Read the model definition and answer for the solid it produces. Units are mm, in the model's axes. A direction names the side the tool comes from. Give positions to 0.01 mm unless a question says otherwise; leave off trailing zeros. Loops run counter-clockwise (first coordinate to the right, second up) from the corner with the lowest first, then second, coordinate; pieces in that order, holes last.
(1) Find section D-D, the plane x = -87. Write down the section's boundary in (y, z), then the cut area to 3 significant figures.
(2) Find section A-A, the plane y = 90.5. Write down the section's boundary in (x, z), then the cut area to 3 significant figures.
(3) Each of these flat-tipped pins is pushed along its axis until it touches: P1, Ø3, axis at x = -18.28, y = 0, coming from the +Z side; P2, Ø0.7, axis at x = -12.5, z = 44.5, coming from the +Y side (3 decimals). Where does it stop, or does it pass through?
(4) Find section B-B, the plane x = 1. Write down the section's boundary in (y, z) (3 decimals), then the cut area to 3 significant figures.
(5) Find section C-C, the plane z = 45.65. State how many separate pieces and enclosed holes the cut face has, then the cut area to 3 significant figures.
(6) Which of the six approach directions +Z, -Z, +X, -X, +Y, -Y give full straight-line access (tool end or side, diameter ignored) to faces 1 (the face through (-38.53, 74.84, 44.87)), 2 (the face through (-35, 2, 43.676)), 3 (the face through (38.53, -74.84, 44.87))?
(7) Straight lines are drawn through the part: probe 1 along Y at (x, z) = (15.24, 44.3) (3 decimals); probe 2 along X at (y, z) = (20, 45.15); probe 3 along Y at (x, z) = (-27, 43.8) (3 decimals). For each, find the intervals that lie inside material, in ascending order.
```python
from build123d import *

# Parameters (mm, degrees)
SKETCH_R        = 2.3622
SKETCH_R_2      = 17.78
PAD_DEPTH       = 2.3622
FILLET_R        = 6.35
FILLET001_R     = 6.35
FILLET002_R     = 6.35
FILLET003_R     = 6.35
FILLET004_R     = 6.35
FILLET005_R     = 3.175
FILLET006_R     = 3.175
FILLET007_R     = 6.35
FILLET008_R     = 6.35
FILLET009_R     = 6.35
FILLET010_R     = 6.35
FILLET011_R     = 6.35
FILLET012_R     = 3.175
FILLET013_R     = 3.175
SKETCH001_R     = 1.651
POCKET_DEPTH    = 2.3632
SKETCH002_R     = 2.2479
POCKET001_DEPTH = 2.3632
SKETCH003_R     = 2.2479
POCKET002_DEPTH = 4.99999


with BuildPart() as part:
    # Sketch (on DatumPlane) → Pad (new body)
    with BuildSketch(Plane.XY.offset(43.6758)):
        Polygon((40.4368, 73.025), (-40.4368, 73.025), (-40.4368, 127), (-65.8368, 127), (-197.6882, 22.225), (-197.6882, -22.225), (-65.8368, -127), (-40.4368, -127), (-40.4368, -73.025), (40.4368, -73.025), (40.4368, -127), (72.1868, -127), (72.1868, 127), (40.4368, 127), align=None)
        with Locations((-21.3868, 66.675)):
            Circle(SKETCH_R, mode=Mode.SUBTRACT)
        with Locations((-21.3868, 53.975)):
            Circle(SKETCH_R, mode=Mode.SUBTRACT)
        with Locations((-21.3868, -53.975)):
            Circle(SKETCH_R, mode=Mode.SUBTRACT)
        with Locations((-21.3868, -66.675)):
            Circle(SKETCH_R, mode=Mode.SUBTRACT)
        with Locations((15.0368, 66.675)):
            Circle(SKETCH_R, mode=Mode.SUBTRACT)
        with Locations((15.24, 53.975)):
            Circle(SKETCH_R, mode=Mode.SUBTRACT)
        with Locations((15.24, -53.975)):
            Circle(SKETCH_R, mode=Mode.SUBTRACT)
        with Locations((15.24, -66.675)):
            Circle(SKETCH_R, mode=Mode.SUBTRACT)
        with Locations((-165.9382, 0)):
            Circle(SKETCH_R_2, mode=Mode.SUBTRACT)
    extrude(amount=PAD_DEPTH)

    # Fillet
    fillet_edges = [part.edges().sort_by_distance(p)[0] for p in [
        (-197.6882, -22.225, 44.8569),
    ]]
    fillet(fillet_edges, radius=FILLET_R)

    # Fillet001
    fillet001_edges = [part.edges().sort_by_distance(p)[0] for p in [
        (-65.8368, -127, 44.8569),
    ]]
    fillet(fillet001_edges, radius=FILLET001_R)

    # Fillet002
    fillet002_edges = [part.edges().sort_by_distance(p)[0] for p in [
        (-40.4368, -127, 44.8569),
    ]]
    fillet(fillet002_edges, radius=FILLET002_R)

    # Fillet003
    fillet003_edges = [part.edges().sort_by_distance(p)[0] for p in [
        (-40.4368, -73.025, 44.8569),
    ]]
    fillet(fillet003_edges, radius=FILLET003_R)

    # Fillet004
    fillet004_edges = [part.edges().sort_by_distance(p)[0] for p in [
        (40.4368, -73.025, 44.8569),
    ]]
    fillet(fillet004_edges, radius=FILLET004_R)

    # Fillet005
    fillet005_edges = [part.edges().sort_by_distance(p)[0] for p in [
        (40.4368, -127, 44.8569),
    ]]
    fillet(fillet005_edges, radius=FILLET005_R)

    # Fillet006
    fillet006_edges = [part.edges().sort_by_distance(p)[0] for p in [
        (72.1868, -127, 44.8569),
    ]]
    fillet(fillet006_edges, radius=FILLET006_R)

    # Fillet007
    fillet007_edges = [part.edges().sort_by_distance(p)[0] for p in [
        (-197.6882, 22.225, 44.8569),
    ]]
    fillet(fillet007_edges, radius=FILLET007_R)

    # Fillet008
    fillet008_edges = [part.edges().sort_by_distance(p)[0] for p in [
        (-65.8368, 127, 44.8569),
    ]]
    fillet(fillet008_edges, radius=FILLET008_R)

    # Fillet009
    fillet009_edges = [part.edges().sort_by_distance(p)[0] for p in [
        (-40.4368, 127, 44.8569),
    ]]
    fillet(fillet009_edges, radius=FILLET009_R)

    # Fillet010
    fillet010_edges = [part.edges().sort_by_distance(p)[0] for p in [
        (40.4368, 73.025, 44.8569),
    ]]
    fillet(fillet010_edges, radius=FILLET010_R)

    # Fillet011
    fillet011_edges = [part.edges().sort_by_distance(p)[0] for p in [
        (-40.4368, 73.025, 44.8569),
    ]]
    fillet(fillet011_edges, radius=FILLET011_R)

    # Fillet012
    fillet012_edges = [part.edges().sort_by_distance(p)[0] for p in [
        (40.4368, 127, 44.8569),
    ]]
    fillet(fillet012_edges, radius=FILLET012_R)

    # Fillet013
    fillet013_edges = [part.edges().sort_by_distance(p)[0] for p in [
        (72.1868, 127, 44.8569),
    ]]
    fillet(fillet013_edges, radius=FILLET013_R)

    # Sketch001 (on Face39 of Fillet013) → Pocket (cut, through all)
    with BuildSketch(Plane.XY.offset(46.038)):
        with Locations((-26.2382, 0)):
            Circle(SKETCH001_R)
        with Locations((-34.2011, 0)):
            Circle(SKETCH001_R)
        with Locations((-26.2382, 9.525)):
            Circle(SKETCH001_R)
        with Locations((-18.2753, 0)):
            Circle(SKETCH001_R)
        with Locations((-26.2382, -9.525)):
            Circle(SKETCH001_R)
    extrude(amount=-POCKET_DEPTH, mode=Mode.SUBTRACT)

    # Sketch002 (on Face44 of Pocket) → Pocket001 (cut, through all)
    with BuildSketch(Plane.XY.offset(46.038)):
        with Locations((-96.923253, -96.214243)):
            Circle(SKETCH002_R)
        with Locations((-72.065864, -115.967033)):
            Circle(SKETCH002_R)
        with Locations((-72.065864, 115.967033)):
            Circle(SKETCH002_R)
        with Locations((-96.923253, 96.214243)):
            Circle(SKETCH002_R)
    extrude(amount=-POCKET001_DEPTH, mode=Mode.SUBTRACT)

    # Sketch003 (on Face48 of Pocket001) → Pocket002 (cut)
    with BuildSketch(Plane.XY.offset(46.038)):
        with Locations((67.4243, -117.475)):
            Circle(SKETCH003_R)
        with Locations((67.4243, -66.675)):
            Circle(SKETCH003_R)
        with Locations((67.4243, 117.475)):
            Circle(SKETCH003_R)
        with Locations((67.4243, 66.675)):
            Circle(SKETCH003_R)
        with Locations((-177.3809, 19.819338)):
            Circle(SKETCH003_R)
        with Locations((-177.3809, -19.819338)):
            Circle(SKETCH003_R)
        with Locations((-143.0528, 0)):
            Circle(SKETCH003_R)
    extrude(amount=-POCKET002_DEPTH, mode=Mode.SUBTRACT)


solid = part.part
```
Entries:
1. outline: (-110.18, 43.68) - (110.18, 43.68) - (110.18, 46.04) - (-110.18, 46.04) - close
1. area: 521 mm2
2. outline: (-111.77, 43.68) - (-40.44, 43.68) - (-40.44, 46.04) - (-111.77, 46.04) - close; (40.44, 43.68) - (72.19, 43.68) - (72.19, 46.04) - (40.44, 46.04) - close
2. area: 244 mm2
3. P1: passes through
3. P2: stops at y = 73.025
4. outline: (-73.025, 43.676) - (73.025, 43.676) - (73.025, 46.038) - (-73.025, 46.038) - close
4. area: 345 mm2
5. separate pieces: 1
5. enclosed holes: 25
5. area: 44,700 mm2
6. face 1: +Z, -Z, +Y
6. face 2: -Z, +X, -X, +Y, -Y
6. face 3: +Z, -Z, -Y
7. probe 1: y = -73.025 to -69.037, -64.313 to -56.337, -51.613 to 51.613, 56.337 to 64.322, 69.028 to 73.025
7. probe 2: x = -197.63 to -179.62, -175.14 to 72.19
7. probe 3: y = -73.025 to -10.99, -8.06 to -1.465, 1.465 to 8.06, 10.99 to 73.025
